For this review, take the finished solid that the model builds, in its own axes (mm). Face numbers are marked on the shaded views. A direction names the side the tool comes from. Give positions to 0.01 mm unless a question says otherwise; leave off trailing zeros. Loops run counter-clockwise (first coordinate to the right, second up) from the corner with the lowest first, then second, coordinate; pieces in that order, holes last.
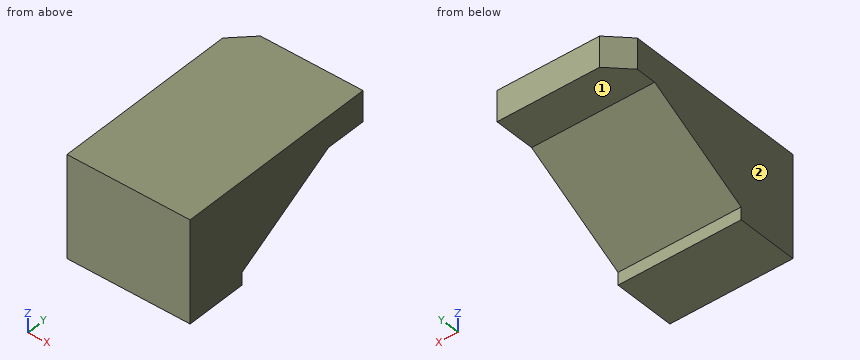
```python
from build123d import *

# Parameters (mm, degrees)
F0_W     = 600
F0_H     = 1000
F1_DEPTH = 500
F3_DEPTH = 600.001
F4_SIZE  = 100


with BuildPart() as f1:
    # F0 (on Top) → F1 (new body)
    with BuildSketch(Plane.XY):
        Rectangle(F0_W, F0_H)
    extrude(amount=F1_DEPTH)

    # F2 (on face) → F3 (cut, through all)
    with BuildSketch(Plane.YZ.offset(300)):
        Polygon((-200, 61.324865), (-200, 0), (500, 0), (500, 350), (300, 350), align=None)
    extrude(amount=-F3_DEPTH, mode=Mode.SUBTRACT)

    # F4
    f4_edges = [f1.edges().sort_by_distance(p)[0] for p in [
        (-300, 500, 425),
    ]]
    chamfer(f4_edges, length=F4_SIZE)


solid = f1.part
```
Item 1: Tool access review of the marked faces 1 and 2: name each direction out of +Z, -Z, +X, -X, +Y, -Y from which nothing blocks a thin tool from reaching the whole face with its end or side.
Answer:
face 1: -Z, +X, -X, +Y
face 2: +Z, -Z, -X, +Y, -Y
Item 2: Take a section at D-D on x = -29.5. Give the boundary of the cut face in (y, z), and give its area (3 significant figures).
Answer:
outline: (-500, 0) - (-200, 0) - (-200, 61.32) - (300, 350) - (500, 350) - (500, 500) - (-500, 500) - close
area: 327,000 mm2
Item 3: Take a section at A-A on x = -240. Give the boundary of the cut face in (y, z), and give its area (3 significant figures).
Answer:
outline: (-500, 0) - (-200, 0) - (-200, 61.32) - (300, 350) - (460, 350) - (460, 500) - (-500, 500) - close
area: 321,000 mm2
Item 4: Clearance check with flat-ended pins moving along their axes: pin 1 Ø8 at (x, z) = (140.5, 65) entering from +Y; pin 2 Ø6 at (x, z) = (-52.5, 226.5) entering from +Y; pin 3 Ø2 at (x, y) = (3.5, 58) entering from -Z. State where each tip first meets the part, or that it passes through.
Answer:
pin 1: stops at y = -186.71
pin 2: stops at y = 91.29
pin 3: stops at z = 209.7
Item 5: Take a section at B-B on y = 412.5. Give the boundary of the cut face in (x, z), and give its area (3 significant figures).
Answer:
outline: (-287.5, 350) - (300, 350) - (300, 500) - (-287.5, 500) - close
area: 88,100 mm2
Item 6: For L1, parallel to Y at x = -5, z = 26; L2, parallel to Z at x = 74, y = 445; L3, parallel to Z at x = -113, y = 249, list the stretches that pass through material, from the lowest coordinate up.
Answer:
L1: y = -500 to -200
L2: z = 350 to 500
L3: z = 320.56 to 500
Item 7: Take a section at C-C on z = 46. Give the boundary of the cut face in (x, y).
Answer:
outline: (-300, -500) - (300, -500) - (300, -200) - (-300, -200) - close
